The listing builds one solid part. Answer for the finished solid, in the listing's coordinates (mm). A direction names the side the tool comes from. Coordinates: 2 decimals unless noted, no trailing zeros. Order: outer loops, then holes, each group sorted by start corner. A loop starts at its lowest first (then second) coordinate and runs counter-clockwise, first axis right, second up. Notation, with made-up numbers: (12.25, 73) -> (50.25, 73) arc R7 cw to (50.25, 80) -> close; hole circle Ø2 at (-25, 50). An arc over 180 degrees is marked (long way). Write each question's results on one line, items separated by ' | '. Start each with the question number.
(1) The part is cut by section A-A, the plane z = 0. Give the vertices of the cut face in (x, y), then the cut area to 3 significant figures.
(2) Determine the mould class of faces 3 (the face through (-17.765, -0.986, -0.228)), 4 (the face through (-25, -1, 0)), 5 (the face through (0, -2, 0)), 6 (the face through (21.235, -0.986, -0.228)) for opening direction X: +X half, -X half, draft (parallel to the pull), parting line (faces both ways), or undercut.
(3) The part is cut by section C-C, the plane x = 0. Give the vertices of the cut face in (y, z), then the cut area to 3 significant figures.
(4) Given pin 1 (10 mm diameter, centred on y = 7, z = 7, fed in from -X); pin 2 (3 mm diameter, centred on y = 7, z = -7, fed in from -X); pin 3 (10 mm diameter, centred on y = 9.5, z = 5.5, fed in from -X); pin 4 (3 mm diameter, centred on x = 19.5, z = 0, fed in from +Y), each flat-ended and moving along its own axis, determine where each tip first touches the part or whether it passes through.
(5) The part is cut by section B-B, the plane x = 19.5. Give the vertices of the cut face in (y, z).
(6) The part is cut by section D-D, the plane z = 4. Give the vertices of the cut face in (x, y).
(7) A tool of negligible diameter and unlimited length cuts with its end or side. For faces 1 (the face through (-11.23, 0, -7.85)), 2 (the face through (0, -1, 15)), from which of +Z, -Z, +X, -X, +Y, -Y can it reach the whole face along a straight path? Write none if from no direction.
(8) Straight lines are drawn through the part: L1, parallel to X at y = -1.2, z = 0; L2, parallel to Y at x = 14, z = -8.25; L3, parallel to Z at x = 19, y = 34. For each, find the intervals that lie inside material, in ascending order.
```python
from build123d import *

# Parameters (mm, degrees)
SKETCH_1_R      = 13.5
SKETCH_1_R_2    = 1.75
EXTRUDE_1_DEPTH = 2
SKETCH_1_3_R    = 13.5
EXTRUDE_2_DEPTH = 16.5


with BuildPart() as part:
    # Sketch 1 → Extrude 1 (new body)
    # profile 1 of 2: a face of its own
    with BuildSketch(Plane(origin=(0, 0, 0), x_dir=(1, 0, 0), z_dir=(0, 1, 0))):
        with BuildLine():
            Line((-22.179487179, -4.803160257), (-7.307692308, -13.099527974))
            ThreePointArc((-7.307692308, -13.099527974), (0, -15), (7.307692308, -13.099527974))
            Line((7.307692308, -13.099527974), (22.179487179, -4.803160257))
            ThreePointArc((22.179487179, -4.803160257), (25, 0), (22.179487179, 4.803160257))
            Line((22.179487179, 4.803160257), (7.307692308, 13.099527974))
            ThreePointArc((7.307692308, 13.099527974), (0, 15), (-7.307692308, 13.099527974))
            Line((-7.307692308, 13.099527974), (-22.179487179, 4.803160257))
            ThreePointArc((-22.179487179, 4.803160257), (-25, 0), (-22.179487179, -4.803160257))
        make_face()
        Circle(SKETCH_1_R, mode=Mode.SUBTRACT)
        with Locations(Location((-19.5, 0, 0), (0, 0, 270))):
            Circle(SKETCH_1_R_2, mode=Mode.SUBTRACT)
        with Locations(Location((19.5, 0, 0), (0, 0, 270))):
            Circle(SKETCH_1_R_2, mode=Mode.SUBTRACT)
    # profile 2 of 2: a face of its own
    with BuildSketch(Plane(origin=(0, 0, 0), x_dir=(1, 0, 0), z_dir=(0, 1, 0))):
        Circle(SKETCH_1_R)
    extrude(amount=-EXTRUDE_1_DEPTH)

    # Sketch 1_3 → Extrude 2 (add)
    with BuildSketch(Plane(origin=(0, 0, 0), x_dir=(1, 0, 0), z_dir=(0, 1, 0))):
        with Locations(Location((0, 0, 0), (0, 0, 270))):
            Circle(SKETCH_1_3_R)
    extrude(amount=EXTRUDE_2_DEPTH)

    # Mirror 3: part across plane


with BuildPart() as part_1:
    add(part.part)
    add(part.part.mirror(Plane.ZX.offset(16.5)))


solid = part_1.part
```
Established:
1) outline: (-25, -2) -> (-21.25, -2) -> (-21.25, 0) -> (-25, 0) -> close; (-25, 33) -> (-21.25, 33) -> (-21.25, 35) -> (-25, 35) -> close; (-17.75, -2) -> (17.75, -2) -> (17.75, 0) -> (13.5, 0) -> (13.5, 33) -> (17.75, 33) -> (17.75, 35) -> (-17.75, 35) -> (-17.75, 33) -> (-13.5, 33) -> (-13.5, 0) -> (-17.75, 0) -> close; (21.25, -2) -> (25, -2) -> (25, 0) -> (21.25, 0) -> close; (21.25, 33) -> (25, 33) -> (25, 35) -> (21.25, 35) -> close | area: 1,060 mm^2
2) face 3: undercut | face 4: -X half | face 5: draft | face 6: undercut
3) outline: (-2, -15) -> (0, -15) -> (0, -13.5) -> (33, -13.5) -> (33, -15) -> (35, -15) -> (35, 15) -> (33, 15) -> (33, 13.5) -> (0, 13.5) -> (0, 15) -> (-2, 15) -> close | area: 1,010 mm^2
4) pin 1: stops at x = -13.35 | pin 2: stops at x = -12.33 | pin 3: stops at x = -13.49 | pin 4: passes through
5) outline: (-2, -6.3) -> (0, -6.3) -> (0, -1.75) -> (-2, -1.75) -> close; (-2, 1.75) -> (0, 1.75) -> (0, 6.3) -> (-2, 6.3) -> close; (33, -6.3) -> (35, -6.3) -> (35, -1.75) -> (33, -1.75) -> close; (33, 1.75) -> (35, 1.75) -> (35, 6.3) -> (33, 6.3) -> close
6) outline: (-23.27, -2) -> (23.27, -2) -> (23.27, 0) -> (12.89, 0) -> (12.89, 33) -> (23.27, 33) -> (23.27, 35) -> (-23.27, 35) -> (-23.27, 33) -> (-12.89, 33) -> (-12.89, 0) -> (-23.27, 0) -> close
7) face 1: none | face 2: +Z, +Y, -Y
8) L1: x = -25 to -21.25, -17.75 to 17.75, 21.25 to 25 | L2: y = -2 to 0, 33 to 35 | L3: z = -6.58 to -1.68, 1.68 to 6.58
